For this review, take the finished solid that the model builds, in its own axes (mm). A direction names the side the tool comes from. Round coordinates to 2 decimals unless told otherwise and drop trailing zeros. Write each loop counter-clockwise with the first axis right and the second up, starting at its lowest first coordinate (ties: lowest second). Pieces come first, ordered by that corner, then holes. Notation, with made-up numbers: M -10.75,28.25 L 45.25,28.25 A14 ccw 45.25,47.25 Z; hole C -10,13 d1. An arc over 180 degrees is marked long. Answer in a Markdown table with one row per item.
```python
from build123d import *

# Parameters (mm, degrees)
SKETCH1_R                = 5
BOSS_EXTRUDE1_DEPTH      = 120
SKETCH2_R                = 3.75
BOSS_EXTRUDE2_DEPTH      = 20
SKETCH3_R                = 3.75
BOSS_EXTRUDE3_DEPTH      = 20
BOSS_EXTRUDE3_DEPTH_BACK = 15
SKETCH4_R                = 1.25
CUT_EXTRUDE1_DEPTH       = 50
SKETCH5_W                = 90
SKETCH5_H                = 25
CUT_EXTRUDE5_DEPTH       = 25
SKETCH6_R                = 5
BOSS_EXTRUDE4_DEPTH      = 5
SKETCH7_R                = 5
BOSS_EXTRUDE5_DEPTH      = 5
SKETCH8_R                = 5
BOSS_EXTRUDE6_DEPTH      = 95
BOSS_EXTRUDE6_DEPTH_BACK = 5
SKETCH9_W                = 90
SKETCH9_H                = 25
BOSS_EXTRUDE7_DEPTH      = 2.5
SKETCH10_R               = 1.25
CUT_EXTRUDE6_DEPTH       = 22.5
CUT_EXTRUDE7_DEPTH       = 120


with BuildPart() as part:
    # Sketch1 → Boss-Extrude1 (new body)
    with BuildSketch(Plane(origin=(0, 0, 0), x_dir=(0, 0, -1), z_dir=(1, 0, 0))):
        Polygon((0, 0), (0, 135), (5, 135), (5, 97), (30, 42.5), (30, 0), align=None)
        with Locations((22.5, 40)):
            Circle(SKETCH1_R, mode=Mode.SUBTRACT)
        with Locations((22.5, 25)):
            Circle(SKETCH1_R, mode=Mode.SUBTRACT)
        Polygon((25, 5), (5, 35), (5, 5), align=None, mode=Mode.SUBTRACT)
    extrude(amount=-BOSS_EXTRUDE1_DEPTH)

    # Sketch2 → Boss-Extrude2 (add)
    with BuildSketch(Plane(origin=(0, 0, -30), x_dir=(-1, 0, 0), z_dir=(0, 0, -1))):
        with Locations((60, 3.75)):
            Circle(SKETCH2_R)
    extrude(amount=BOSS_EXTRUDE2_DEPTH)

    # Sketch3 → Boss-Extrude3 (add, two sides)
    with BuildSketch(Plane(origin=(0, 0, -30), x_dir=(-1, 0, 0), z_dir=(0, 0, -1))) as boss_extrude3_sk:
        with Locations((60, 52.25)):
            Circle(SKETCH3_R)
    extrude(amount=BOSS_EXTRUDE3_DEPTH)
    extrude(boss_extrude3_sk.sketch, amount=-BOSS_EXTRUDE3_DEPTH_BACK)

    # Sketch4 → Cut-Extrude1 (cut)
    with BuildSketch(Plane.XY):
        with Locations((-60, 15)):
            Circle(SKETCH4_R)
    extrude(amount=-CUT_EXTRUDE1_DEPTH, mode=Mode.SUBTRACT)

    # Sketch5 → Cut-Extrude5 (cut)
    with BuildSketch(Plane(origin=(0, 0, -30), x_dir=(-1, 0, 0), z_dir=(0, 0, -1))):
        with Locations((60, 23.5)):
            Rectangle(SKETCH5_W, SKETCH5_H)
    extrude(amount=-CUT_EXTRUDE5_DEPTH, mode=Mode.SUBTRACT)

    # Sketch6 → Boss-Extrude4 (add)
    with BuildSketch(Plane.ZY.offset(15)):
        with Locations((-22.5, 25)):
            Circle(SKETCH6_R)
    extrude(amount=-BOSS_EXTRUDE4_DEPTH)

    # Sketch7 → Boss-Extrude5 (add)
    with BuildSketch(Plane(origin=(-105, 0, 0), x_dir=(0, 0, -1), z_dir=(1, 0, 0))):
        with Locations((22.5, 25)):
            Circle(SKETCH7_R)
    extrude(amount=-BOSS_EXTRUDE5_DEPTH)

    # Sketch8 → Boss-Extrude6 (add, two sides)
    with BuildSketch(Plane.ZY.offset(15)) as boss_extrude6_sk:
        with Locations((-22.5, 40)):
            Circle(SKETCH8_R)
    extrude(amount=BOSS_EXTRUDE6_DEPTH)
    extrude(boss_extrude6_sk.sketch, amount=-BOSS_EXTRUDE6_DEPTH_BACK)

    # Sketch9 → Boss-Extrude7 (add)
    with BuildSketch(Plane.XZ.offset(-36)):
        with Locations((-60, -17.5)):
            Rectangle(SKETCH9_W, SKETCH9_H)
    extrude(amount=BOSS_EXTRUDE7_DEPTH)

    # Sketch10 → Cut-Extrude6 (cut)
    with BuildSketch(Plane.XY):
        with Locations((-110, 115)):
            Circle(SKETCH10_R)
        with Locations((-10, 115)):
            Circle(SKETCH10_R)
    extrude(amount=-CUT_EXTRUDE6_DEPTH, mode=Mode.SUBTRACT)

    # Sketch11 → Cut-Extrude7 (cut)
    with BuildSketch(Plane(origin=(0, 0, 0), x_dir=(0, 0, -1), z_dir=(1, 0, 0))):
        Polygon((5, 85.00791928), (5, 50.00791928), (21.055045872, 50.00791928), align=None)
    extrude(amount=-CUT_EXTRUDE7_DEPTH, mode=Mode.SUBTRACT)


solid = part.part
```
Q1. Take a section at A-A (y = 40). State the section outline as (x, z) points.
Found:
| item | result |
|---|---|
| outline | M -120,-30 L 0,-30 L 0,-27.5 L -10,-27.5 L -10,-17.5 L 0,-17.5 L 0,0 L -120,0 L -120,-17.5 L -110,-17.5 L -110,-27.5 L -120,-27.5 Z |
Q2. Take a section at C-C (x = -107). State the section outline as (y, z) points.
Found:
| item | result |
|---|---|
| outline | M 0,-30 L 42.5,-30 L 97,-5 L 135,-5 L 135,0 L 0,0 Z; hole M 5,-25 L 35,-5 L 5,-5 Z; hole M 50.01,-21.06 L 85.01,-5 L 50.01,-5 Z |
Q3. Insertion check: P1, Ø13, axis at x = -76.5, y = 12.5, coming from the -Z side; P2, Ø1.5, axis at x = -10, y = 115, coming from the -Z side; P3, Ø10, axis at x = -56, z = -23.5, coming from the +Y side; P4, Ø5, axis at y = 23.5, z = -23.5, coming from the -X side. Each pin has a flat end and moves straight along its axis. Give the tip position at first contact, or say it passes through.
Found:
| item | result |
|---|---|
| P1 | z = -30 |
| P2 | through |
| P3 | y = 67.57 |
| P4 | x = -110 |
Q4. Take a section at B-B (z = -33). State the section outline as (x, y) points, then the cut area to 3 significant figures.
Found:
| item | result |
|---|---|
| outline | C -60,3.75 d7.5; C -60,52.25 d7.5 |
| area | 88.4 mm² |
Q5. For probe 1 along X at (y, z) = (115, -2.65); probe 2 along X at (y, z) = (19.5, -19); probe 3 along Y at (x, z) = (-10, -1.6), list the stretches that pass through material, from the lowest coordinate up.
Found:
| item | result |
|---|---|
| probe 1 | -120 to -111.25, -108.75 to -11.25, -8.75 to 0 |
| probe 2 | -120 to -105, -15 to 0 |
| probe 3 | 0 to 113.75, 116.25 to 135 |
Q6. Mouldability with a two-part tool opening along Z and no side actions: class faces 4 (the face through (-59, 68, -5)), 5 (the face through (-61, 36, -30)), 6 (the face through (-15, 25, -21)), 7 (the face through (-59, 67, 0)) as +Z half, -Z half, draft (parallel to the pull), parting line (faces both ways), or undercut.
Found:
| item | result |
|---|---|
| face 4 | undercut |
| face 5 | -Z half |
| face 6 | draft |
| face 7 | +Z half |
Q7. Machinability: for faces 1 (the face through (-63.577, 4.876, -39.86)), 2 (the face through (-10, 25, -23)), 3 (the face through (-59.16, 67.26, -13.14)), which of the approach directions +Z, -Z, +X, -X, +Y, -Y give a long, thin tool a straight path to every point of the face, cutting with its end or side? Answer none if there is none.
Found:
| item | result |
|---|---|
| face 1 | -Z |
| face 2 | +X |
| face 3 | +X, -X |
Q8. Take a section at D-D (y = 9). State the section outline as (x, z) points, then the cut area to 3 significant figures.
Found:
| item | result |
|---|---|
| outline | M -120,-30 L 0,-30 L 0,-22.33 L -120,-22.33 Z; M -120,-5 L 0,-5 L 0,0 L -120,0 Z |
| area | 1,520 mm² |
